Part model, mm, in its own coordinate system. A direction names the side the tool comes from. Round coordinates to 2 decimals unless told otherwise and drop trailing zeros. Loops run counter-clockwise (first coordinate to the right, second up) from the corner with the lowest first, then second, coordinate; pieces in that order, holes last. Notation, with made-up numbers: M 8,-32.5 L 43,-32.5 A16 ccw 43,-5.5 Z; hole C 2,79.25 d8. An arc over 180 degrees is marked long. Write each question's results on one line, items separated by ' | '.
Autodesk Inventor part; units mm, degrees
ref_plane "YZ Plane" through (0, 0, 0) normal (1, 0, 0) x (0, 1, 0)
ref_plane "XZ Plane" through (0, 0, 0) normal (0, 1, 0) x (-1, 0, 0)
ref_plane "XY Plane" through (0, 0, 0) normal (0, 0, 1) x (1, 0, 0)
sketch "Sketch1" plane through (0, 0, 0) normal (0, 0, 1) x (1, 0, 0)
  line L0 (4, 3) -> (6, 3)
  line L1 (6, 3) -> (6, 3)
  line L2 (16.5, 3.5) -> (16.5, 3.5)
  line L3 (35, 3) -> (35, 0)
  line L4 (4, 3) -> (4, 2.5)
  line L5 (4, 2.5) -> (1, 2.5)
  line L6 (1, 2.5) -> (1, 0)
  line L7 (1, 0) -> (35, 0)
  line L8 (23, 3) -> (35, 3)
  line L9 (23, 3.5) -> (17, 3.5)
  line L10 (23, 3.5) -> (23, 3)
  line L11 (17, 3.5) -> (17, 4)
  line L12 (17, 4) -> (16, 4)
  line L13 (16, 4) -> (16, 3)
  line L14 (6, 3) -> (16, 3)
  point P0 (0, 0)
  dimension "d1" = 2
  dimension "d25" = 3
  dimension "d26" = 2.5
  dimension "d40" = 12
  dimension "d41" = 3
  dimension "d42" = 0.5
  dimension "d44" = 6
  dimension "d45" = 1
  dimension "d46" = 10
  dimension "d47" = 3
  dimension "d48" = 3
revolve "Revolution2" add sketch "Sketch1" angle 360 about axis through (1, 0, 0) along (1, 0, 0)
sketch "Sketch3" plane through (35, 0, 0) normal (1, 0, 0) x (0, 0, -1)
  circle A0 centre (0, 0) radius 3
  line L0 (-1.6583, 2.5) -> (1.6583, 2.5)
  line L1 (-1.6583, -2.5) -> (1.6583, -2.5)
  point P0 (0, 0)
  dimension "d21" = 0.5
  dimension "d31" = 0.5
extrude "Extrusion2" [suppressed]
sketch "Sketch4" plane through (4, 0, 0) normal (-1, 0, 0) x (0, 0, 1)
  line L0 (-1.6583, 2.5) -> (1.6583, 2.5)
  circle A0 centre (0, 0) radius 3
  line L1 (-1.6583, -2.5) -> (1.6583, -2.5)
  point P0 (0, 0)
  dimension "d27" = 0.5
  dimension "d30" = 0.5
extrude "Extrusion3" [suppressed]
sketch "Sketch5" plane through (35, 0, 0) normal (1, 0, 0) x (0, 0, -1)
  point P0 (0, 0)
  point P1 (0, 0)
hole "Hole1" at (35, 0, 0) direction (-1, 0, 0) diameter 2.459 depth 10 tip angle 118
sketch "Sketch6" plane through (35, 0, 0) normal (1, 0, 0) x (0, 0, -1)
  circle A0 centre (0, 0) radius 1.2295
  circle A1 centre (0, 0) radius 3
  circle A2 centre (0, 0) radius 3
  line L0 (-2.0396, 2.2) -> (2.0396, 2.2)
  line L1 (-2.0396, -2.2) -> (2.0396, -2.2)
  dimension "d56" = 2.2
  dimension "d57" = 2.2
extrude "Extrusion4" cut sketch "Sketch6" against normal up to surface (12 mm away) contours L0 A1 | A1 L1
properties part number "Wał koła" material "Aluminum 6061, Welded"
Item 1: Which spindle directions (+Z, -Z, +X, -X, +Y, -Y) get a long thin tool onto all of the face, cutting with end or side? Do faces 5 (the cylindrical face through (29, 0, 3)), 6 (the cylindrical face through (29, 0, -3)), 7 (the cylindrical face through (16.493, -0.867, 3.905)), 8 (the flat face through (29, 2.2, 0)), 9 (the cylindrical face through (10, -3, 0)). Say none if no direction does.
Filled sheet:
face 5: +Z, +X | face 6: -Z, +X | face 7: +X, -X | face 8: +Z, -Z, +X, +Y | face 9: -X
Item 2: Band-saw the part on C-C on x = 13. Give the cut face in (y, z), and give its area (3 significant figures).
Filled sheet:
outline: C 0,0 d6 | area: 28.3 mm^2
Item 3: Two-plate mould, pull along Y, no slides. Class faces 1 (the cylindrical face through (29.93, 0.748, 0.976)), 2 (the flat face through (29, -2.2, 0)), 3 (the conical face through (24.39, -0.21, 0.05)), 4 (the cylindrical face through (19.958, 3.233, 1.341)): +Y half, -Y half, draft (parallel to the pull), parting line (faces both ways), or undercut.
Filled sheet:
face 1: undercut | face 2: -Y half | face 3: undercut | face 4: parting line
Item 4: Band-saw the part on B-B on x = 19. Give the cut face in (y, z), and give its area (3 significant figures).
Filled sheet:
outline: C 0,0 d7 | area: 38.5 mm^2
Item 5: Wall check: L1, parallel to Z at x = 28, y = 0; L2, parallel to Y at x = 28, z = 0; L3, parallel to X at y = 0, z = 3.75. Give the ranges that are in metal, low to high.
Filled sheet:
L1: -3 to -1.23, 1.23 to 3 | L2: -2.2 to -1.23, 1.23 to 2.2 | L3: 16 to 17
Item 6: Drop flat-ended pins along their axis: P1, Ø3.5, axis at x = 26, z = 1, coming from the +Y side; P2, Ø1, axis at y = -3, z = -1, coming from the -X side; P3, Ø2, axis at x = 19, y = 0, coming from the +Z side. Give the stop position or say it passes through.
Filled sheet:
P1: y = 2.2 | P2: x = 4 | P3: z = 3.5
Item 7: Band-saw the part on A-A on x = 31. Give the cut face in (y, z), and give its area (3 significant figures).
Filled sheet:
outline: M -2.2,-2.04 A3 ccw 2.2,-2.04 L 2.2,2.04 A3 ccw -2.2,2.04 Z; hole C 0,0 d2.46 | area: 19.0 mm^2
